Input: dimensioned drawing with shaded views. Units: mm. Origin: part minimum x, y, z. Give positions to 0.01 mm unless a question says otherwise; leave off trailing zeros. Order: outer loops, then holes, each group sorted by start corner. A loop starts at its lowest first (then second) coordinate and runs counter-clockwise, first axis right, second up. Notation, with made-up numbers: (26, 30) -> (78, 30) arc R14 cw to (78, 37) -> close; hole circle Ø7 at (-32, 48.5). An arc over 180 degrees is marked (long way). Use CSV: the item, a comma, the result in double quotes.
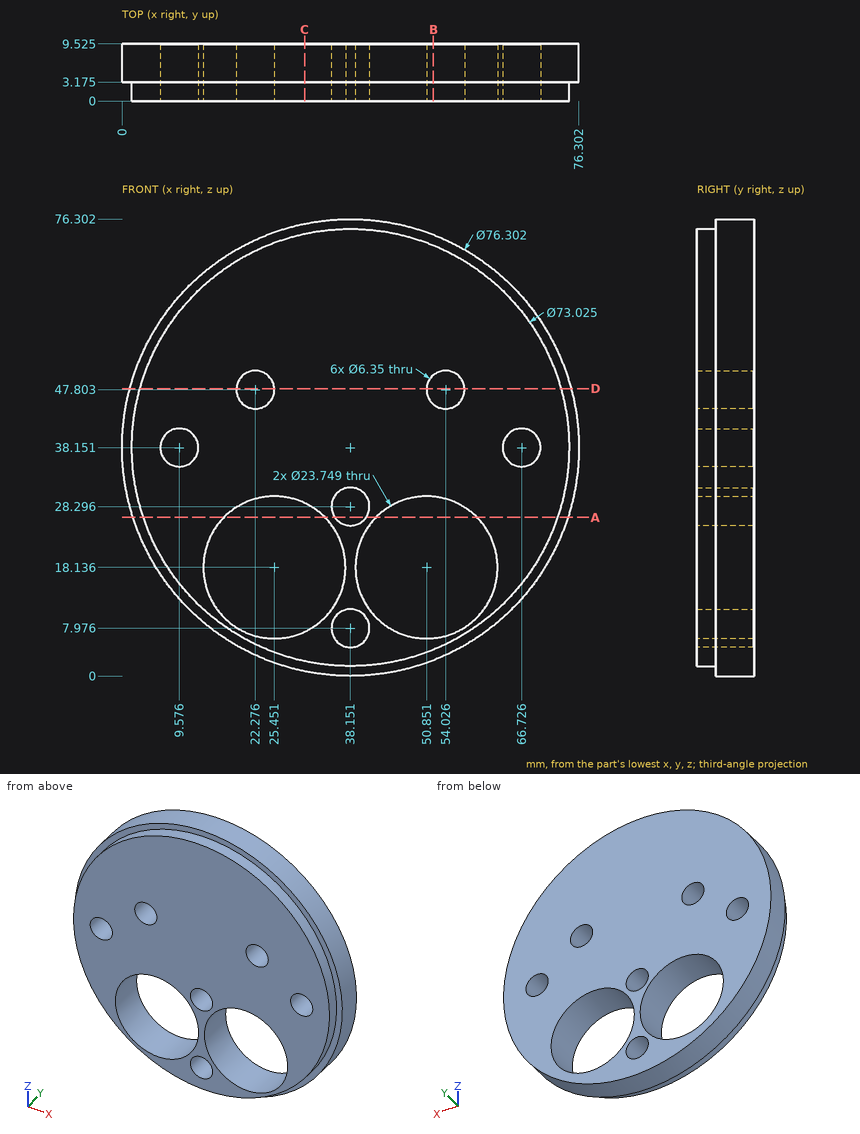
1. Section query B-B on x = 52. Return loops of the section in (y, z) (1 decimal).
Answer below:
outline,"(0, 4.4) -> (3.2, 4.4) -> (3.2, 2.6) -> (9.5, 2.6) -> (9.5, 6.3) -> (0, 6.3) -> close; (0, 30) -> (9.5, 30) -> (9.5, 45.4) -> (0, 45.4) -> close; (0, 50.2) -> (9.5, 50.2) -> (9.5, 73.7) -> (3.2, 73.7) -> (3.2, 71.9) -> (0, 71.9) -> close"
2. Section query A-A on z = 26.5. Return loops of the section in (x, y) (1 decimal), plus the area to 3 significant figures.
Answer below:
outline,"(1.8, 3.2) -> (3.5, 3.2) -> (3.5, 0) -> (17, 0) -> (17, 9.5) -> (1.8, 9.5) -> close; (33.9, 0) -> (35.5, 0) -> (35.5, 9.5) -> (33.9, 9.5) -> close; (40.8, 0) -> (42.4, 0) -> (42.4, 9.5) -> (40.8, 9.5) -> close; (59.3, 0) -> (72.8, 0) -> (72.8, 3.2) -> (74.5, 3.2) -> (74.5, 9.5) -> (59.3, 9.5) -> close"
area,"310 mm²"
3. Ray query, line 1 along X through (y, z) = (8.5, 20) (1 decimal); line 2 along X through (y, z) = (4, 14.5) (1 decimal); line 3 along Z through (x, y) = (59, 8). Return the intervals inside material, ascending.
Answer below:
line 1,"x = 4.6 to 13.7, 37.2 to 39.1, 62.6 to 71.7"
line 2,"x = 8.2 to 14.1, 36.8 to 39.5, 62.2 to 68.1"
line 3,"z = 6.2 to 9.5, 26.77 to 70.1"
4. Section query C-C on x = 30.5. Return loops of the section in (y, z) (1 decimal).
Answer below:
outline,"(0, 2.4) -> (3.2, 2.4) -> (3.2, 0.8) -> (9.5, 0.8) -> (9.5, 7.4) -> (0, 7.4) -> close; (0, 28.9) -> (9.5, 28.9) -> (9.5, 75.5) -> (3.2, 75.5) -> (3.2, 73.9) -> (0, 73.9) -> close"
5. Pin query (flat end, axial travel): P1, Ø4, axis at x = 54.03, z = 47.8, coming from the +Y side; P2, Ø4, axis at y = 1.5, z = 51, coming from the -X side; P3, Ø12, axis at x = 22, z = 9, coming from the -Y side; P4, Ø1, axis at x = 24, y = 6.5, coming from the -Z side (1 decimal). Return the tip coordinate at first contact, or that it passes through.
Answer below:
P1,"passes through"
P2,"stops at x = 1.86"
P3,"stops at y = 0"
P4,"stops at z = 2.5"
6. Section query D-D on z = 48. Return loops of the section in (x, y) (1 decimal).
Answer below:
outline,"(1.3, 3.2) -> (3, 3.2) -> (3, 0) -> (19.1, 0) -> (19.1, 9.5) -> (1.3, 9.5) -> close; (25.4, 0) -> (50.9, 0) -> (50.9, 9.5) -> (25.4, 9.5) -> close; (57.2, 0) -> (73.3, 0) -> (73.3, 3.2) -> (75, 3.2) -> (75, 9.5) -> (57.2, 9.5) -> close"
